```python
from build123d import *

# Parameters (mm, degrees)
SKETCH1_R              = 6.35
BOSS_EXTRUDE1_DEPTH    = 125.4125
SKETCH2_R              = 1.89611
CUT_EXTRUDE1_DEPTH     = 3.175
CUT_EXTRUDE2_START     = 3.175
CUT_EXTRUDE2_OUTLINE_R = 1.89611
CUT_EXTRUDE2_DEPTH     = 3.1750001
SKETCH3_OUTSIDE_W      = 40.038
SKETCH3_OUTSIDE_H      = 40.038
SKETCH3_OUTSIDE_R      = 3.175
CUT_EXTRUDE3_DEPTH     = 12.7
SKETCH4_R              = 3.96875
BOSS_EXTRUDE2_DEPTH    = 6.35


# Read off the part's stored shape, not the designer's step: Cut-Extrude2
with BuildPart() as part:
    # Sketch1 → Boss-Extrude1 (new body)
    with BuildSketch(Plane(origin=(0, 0, 0), x_dir=(0, 0, -1), z_dir=(1, 0, 0))):
        with Locations((6.35, 0)):
            Circle(SKETCH1_R)
    extrude(amount=BOSS_EXTRUDE1_DEPTH)

    # Sketch2 → Cut-Extrude1 (cut)
    with BuildSketch(Plane.XY):
        with Locations((13.24991, 0)):
            Circle(SKETCH2_R)
    extrude(amount=-CUT_EXTRUDE1_DEPTH, mode=Mode.SUBTRACT)

    # Cut-Extrude2 outline → Cut-Extrude2 (cut)
    with BuildSketch(Plane(origin=(0, 0, 0), x_dir=(1, 0, 0), z_dir=(0, 1, 0)).offset(CUT_EXTRUDE2_START)):
        with Locations((13.23805984, 6.910255895)):
            Circle(CUT_EXTRUDE2_OUTLINE_R)
    extrude(amount=CUT_EXTRUDE2_DEPTH, mode=Mode.SUBTRACT)

    # Sketch3 outside → Cut-Extrude3 (cut)
    with BuildSketch(Plane(origin=(125.4125, 0, 0), x_dir=(0, 0, -1), z_dir=(1, 0, 0))):
        with Locations((6.35, 0)):
            Rectangle(SKETCH3_OUTSIDE_W, SKETCH3_OUTSIDE_H)
        with Locations((6.35, 0)):
            Circle(SKETCH3_OUTSIDE_R, mode=Mode.SUBTRACT)
    extrude(amount=-CUT_EXTRUDE3_DEPTH, mode=Mode.SUBTRACT)

    # Sketch4 → Boss-Extrude2 (add)
    with BuildSketch(Plane(origin=(112.7125, 0, 0), x_dir=(0, 0, -1), z_dir=(1, 0, 0))):
        with Locations((6.35, 0)):
            Circle(SKETCH4_R)
    extrude(amount=BOSS_EXTRUDE2_DEPTH)


solid = part.part
```
Model file for the job. Use its own axes, mm. A direction names the side the tool comes from. Give positions to 0.01 mm unless a question says otherwise; leave off trailing zeros. Loops run counter-clockwise (first coordinate to the right, second up) from the corner with the lowest first, then second, coordinate; pieces in that order, holes last. Notation, with made-up numbers: (75, -3) - (86, -3) arc R36 cw to (86, 35) - close; hole circle Ø7 at (21, 50.5). An arc over 180 degrees is marked (long way). One line per item, written item: value. Start each with the question number.
1. Slice it at A-A (y = 0). List the corners of the cut face in (x, z) (1 decimal), plus the area to 3 significant figures.
2. Probe L1, parallel to X at y = 0, z = -0.75; L2, parallel to X at y = -3.25, z = -2.5; L3, parallel to Z at x = 59.5, y = 0.5. List the from-to ranges inside material, lowest first. Write a range as from..to.
3. Pin check, flat tips, straight feed: pin 1 (6 mm diameter, centred on x = 13.24, z = -6.91, fed in from -Y); pin 2 (3 mm diameter, centred on x = 13.25, y = 0, fed in from +Z) (3 decimals); pin 3 (2 mm diameter, centred on x = 87.5, y = -2.5, fed in from -Z); pin 4 (4 mm diameter, centred on x = 51, y = -4, fed in from -Z). Stop position of each tip, or through.
4. Slice it at B-B (x = 27). List the corners of the cut face in (y, z), plus the area to 3 significant figures.
5. Pull direction Y, two halves, no side cores. Call faces 4 (the flat face through (112.712, -3, -3)), 5 (the cylindrical face through (115.843, 1.192, -10.135)), 6 (the flat face through (13, 0, -3.175)), 7 (the cylindrical face through (11.356, 0.083, -1.565)): pulls with the +Y half, pulls with the -Y half, needs draft (parallel to the pull), parting line crosses it, or undercut.
6. Which spindle directions (+Z, -Z, +X, -X, +Y, -Y) get a long thin tool onto all of the face, cutting with end or side? Do faces 1 (the flat face through (125.412, 0, -6)), 2 (the cylindrical face through (14.113, 4.741, -5.228)), 3 (the cylindrical face through (122.28, 0.14, -3.18)). Say none if no direction does.
Solution:
1. outline: (0, -12.7) - (112.7, -12.7) - (112.7, -10.3) - (119.1, -10.3) - (119.1, -9.5) - (125.4, -9.5) - (125.4, -3.2) - (119.1, -3.2) - (119.1, -2.4) - (112.7, -2.4) - (112.7, 0) - (15.1, 0) - (15.1, -3.2) - (11.4, -3.2) - (11.4, 0) - (0, 0) - close
1. area: 1,510 mm^2
2. L1: x = 0..11.35, 15.15..112.71
2. L2: x = 0..112.71
2. L3: z = -12.68..-0.02
3. pin 1: stops at y = -6.35
3. pin 2: stops at z = -3.175
3. pin 3: stops at z = -12.52
3. pin 4: stops at z = -12.38
4. outline: circle Ø12.7 at (0, -6.35)
4. area: 127 mm^2
5. face 4: needs draft
5. face 5: parting line crosses it
5. face 6: undercut
5. face 7: undercut
6. face 1: +Z, -Z, +X, +Y, -Y
6. face 2: +Y
6. face 3: +X
